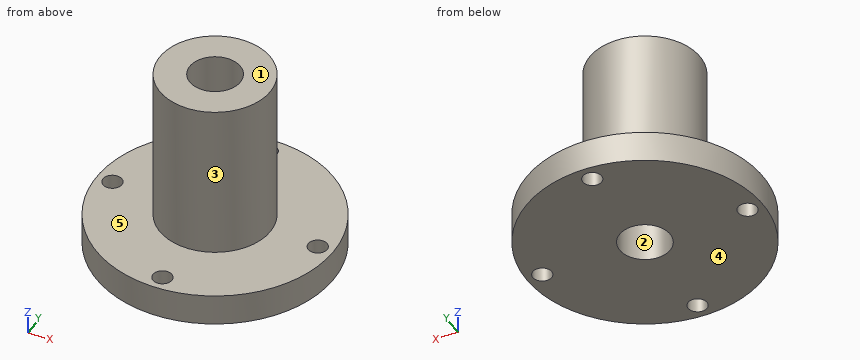
```python
from build123d import *

# Parameters (mm, degrees)
SKETCH_1_R          = 37.5
EXTRUDE_1_DEPTH     = 10
SKETCH_2_R          = 17.5
EXTRUDE_2_DEPTH     = 50
SKETCH_3_R          = 8
CUT_EXTRUDE_1_DEPTH = 61
SKETCH_4_R          = 3
CUT_EXTRUDE_2_DEPTH = 10


with BuildPart() as part:
    # 草图1 → 凸台-拉伸1 (new body)
    with BuildSketch(Plane.XY):
        Circle(SKETCH_1_R)
    extrude(amount=EXTRUDE_1_DEPTH)

    # 草图2 → 凸台-拉伸2 (add)
    with BuildSketch(Plane.XY.offset(10)):
        Circle(SKETCH_2_R)
    extrude(amount=EXTRUDE_2_DEPTH)

    # 草图3 → 切除-拉伸1 (cut, through all)
    with BuildSketch(Plane.XY.offset(60)):
        Circle(SKETCH_3_R)
    extrude(amount=-CUT_EXTRUDE_1_DEPTH, mode=Mode.SUBTRACT)

    # 草图4 → 切除-拉伸2 (cut)
    with BuildSketch(Plane.XY.offset(10)):
        with Locations((0, 32.5)):
            Circle(SKETCH_4_R)
        with Locations((32.5, 0)):
            Circle(SKETCH_4_R)
        with Locations((0, -32.5)):
            Circle(SKETCH_4_R)
        with Locations((-32.5, 0)):
            Circle(SKETCH_4_R)
    extrude(amount=-CUT_EXTRUDE_2_DEPTH, mode=Mode.SUBTRACT)


solid = part.part
```
For this review, take the finished solid that the model builds, in its own axes (mm). Face numbers are marked on the shaded views. A direction names the side the tool comes from. Round coordinates to 2 decimals unless told otherwise and drop trailing zeros. Loops run counter-clockwise (first coordinate to the right, second up) from the corner with the lowest first, then second, coordinate; pieces in that order, holes last.
Q1. Mouldability with a two-part tool opening along X and no side actions: class the marked faces 1, 2 and 3 as +X half, -X half, draft (parallel to the pull), parting line (faces both ways), or undercut.
Result sheet:
face 1: draft
face 2: undercut
face 3: parting line
Q2. Add section C-C on z = 38. Write out the cut boundary in (x, y), plus the area to 3 significant figures.
Result sheet:
outline: circle Ø35 at (0, 0); hole circle Ø16 at (0, 0)
area: 761 mm2
Q3. Add section A-A on y = 0. Write out the cut boundary in (x, z), plus the area to 3 significant figures.
Result sheet:
outline: (-37.5, 0) - (-35.5, 0) - (-35.5, 10) - (-37.5, 10) - close; (-29.5, 0) - (-8, 0) - (-8, 60) - (-17.5, 60) - (-17.5, 10) - (-29.5, 10) - close; (8, 0) - (29.5, 0) - (29.5, 10) - (17.5, 10) - (17.5, 60) - (8, 60) - close; (35.5, 0) - (37.5, 0) - (37.5, 10) - (35.5, 10) - close
area: 1,420 mm2
Q4. To check wall thickness, follow line 1 along Y through (x, z) = (0, 6); line 2 along Y through (x, z) = (0, 23); line 3 along Z through (x, y) = (7, -33.5). State the ranges of each line that lie inside material, in increasing order.
Result sheet:
line 1: y = -37.5 to -35.5, -29.5 to -8, 8 to 29.5, 35.5 to 37.5
line 2: y = -17.5 to -8, 8 to 17.5
line 3: z = 0 to 10
Q5. Machinability: for the marked faces 4 and 5, which of the approach directions +Z, -Z, +X, -X, +Y, -Y give a long, thin tool a straight path to every point of the face, cutting with its end or side? Answer none if there is none.
Result sheet:
face 4: -Z, +X, -X, +Y, -Y
face 5: +Z
Q6. Insertion check: pin 1 Ø8 at (x, z) = (7.5, 24.5) entering from +Y; pin 2 Ø1.5 at (x, z) = (5, 18) entering from +Y; pin 3 Ø5 at (y, z) = (1, 25.5) entering from +X. Each pin has a flat end and moves straight along its axis. Give the tip position at first contact, or say it passes through.
Result sheet:
pin 1: stops at y = 17.15
pin 2: stops at y = 16.98
pin 3: stops at x = 17.5
Q7. Add section D-D on x = 32.5. Write out the cut boundary in (y, z), plus the area to 3 significant figures.
Result sheet:
outline: (-18.71, 0) - (-3, 0) - (-3, 10) - (-18.71, 10) - close; (3, 0) - (18.71, 0) - (18.71, 10) - (3, 10) - close
area: 314 mm2
